from build123d import *

# Parameters (mm, degrees)
ESQUISSE1_R             = 8
BOSS_EXTRU_1_DEPTH      = 47.9
ESQUISSE2_R             = 4
BOSS_EXTRU_2_DEPTH      = 2.8
ESQUISSE3_R             = 2
BOSS_EXTRU_3_DEPTH      = 10
ESQUISSE5_W             = 4
ESQUISSE5_H             = 8
ENL_V_MAT_EXTRU_1_DEPTH = 10
BOSS_EXTRU_4_START      = 1.5
ESQUISSE6_R             = 4
BOSS_EXTRU_4_DEPTH      = 1.5
ESQUISSE7_R             = 1
ENL_V_MAT_EXTRU_2_DEPTH = 6


with BuildPart() as part:
    # Esquisse1 → Boss.-Extru.1 (new body)
    with BuildSketch(Plane.XY):
        Circle(ESQUISSE1_R)
    extrude(amount=BOSS_EXTRU_1_DEPTH)

    # Esquisse2 → Boss.-Extru.2 (add)
    with BuildSketch(Plane.XY.offset(47.9)):
        Circle(ESQUISSE2_R)
    extrude(amount=BOSS_EXTRU_2_DEPTH)

    # Esquisse3 → Boss.-Extru.3 (add)
    with BuildSketch(Plane.XY.offset(50.7)):
        Circle(ESQUISSE3_R)
    extrude(amount=BOSS_EXTRU_3_DEPTH)

    # Esquisse5 → Enlèv. mat.-Extru.1 (cut)
    with BuildSketch(Plane(origin=(0, 1, 0), x_dir=(1, 0, 0), z_dir=(0, 1, 0))):
        with Locations((0, -56.7)):
            Rectangle(ESQUISSE5_W, ESQUISSE5_H)
    extrude(amount=ENL_V_MAT_EXTRU_1_DEPTH, mode=Mode.SUBTRACT)

    # Esquisse6 → Boss.-Extru.4 (add)
    with BuildSketch(Plane(origin=(0, 0, 0), x_dir=(-1, 0, 0), z_dir=(0, 0, -1)).offset(BOSS_EXTRU_4_START)):
        with Locations(Location((0, 0, 0), (0, 0, 180))):
            Circle(ESQUISSE6_R)
    extrude(amount=-BOSS_EXTRU_4_DEPTH)

    # Esquisse7 → Enlèv. mat.-Extru.2 (cut)
    with BuildSketch(Plane.XY.offset(47.9)):
        with Locations((6, 0)):
            Circle(ESQUISSE7_R)
        with Locations((-6, 0)):
            Circle(ESQUISSE7_R)
    extrude(amount=-ENL_V_MAT_EXTRU_2_DEPTH, mode=Mode.SUBTRACT)


solid = part.part
Geometry check sheet. Reference: the model listing, model coordinates, mm. A direction names the side the tool comes from. Coordinates: 2 decimals unless noted, no trailing zeros. Order: outer loops, then holes, each group sorted by start corner. A loop starts at its lowest first (then second) coordinate and runs counter-clockwise, first axis right, second up. Notation, with made-up numbers: (15.25, 16.5) -> (21.25, 16.5) arc R18 cw to (21.25, 32.5) -> close; hole circle Ø11 at (39, -28.75). An arc over 180 degrees is marked (long way). Use a Markdown table: item, result. Add a question column.
1. Cross-section at A-A (x = 0). Enter the section's corners in (y, z), and give its area (3 significant figures).
2. Go/stop test with flat-tipped pins: pin 1 Ø2.5 at (x, y) = (-6, 0) entering from -Z; pin 2 Ø1.6 at (x, y) = (6, -0.5) entering from +Z; pin 3 Ø4 at (y, z) = (-2.5, 45) entering from -X. Record where each tip stops, or that it passes through.
3. Set-up check for faces 1 (the face through (-4, -2, 0)), 2 (the face through (-0.867, -3.905, 49.28)), 3 (the face through (0, 1, 57)): record each of +Z, -Z, +X, -X, +Y, -Y from which the full face is reachable in a straight line by a thin tool's end or side.
4. Material ranges on L1, parallel to X at y = -0.25, z = 8; L2, parallel to Y at x = -6, z = 46.3; L3, parallel to Z at x = -2, y = -3, recorded low to high.
5. Cross-section at B-B (y = 0). Enter the section's corners in (x, z), and give its area (3 significant figures).
6. Cross-section at D-D (z = 30.5). Enter the section's corners in (x, y), and give its area (3 significant figures).
7. Cross-section at C-C (z = 44.5). Enter the section's corners in (x, y), and give its area (3 significant figures).
8. Mould release check, pull along Y, two halves, no side actions. Record for faces 4 (the face through (-1.73, -7.81, 23.61)), 5 (the face through (-6.8, -0.6, 44.9)), 6 (the face through (0, 0, 60.7)): pulls with the +Y half, pulls with the -Y half, needs draft (parallel to the pull), parting line crosses it, or undercut.
Filled sheet:
| question | item | result |
|---|---|---|
| 1 | outline | (-8, 0) -> (-4, 0) -> (-4, -1.5) -> (4, -1.5) -> (4, 0) -> (8, 0) -> (8, 47.9) -> (4, 47.9) -> (4, 50.7) -> (2, 50.7) -> (2, 52.7) -> (1, 52.7) -> (1, 60.7) -> (-2, 60.7) -> (-2, 50.7) -> (-4, 50.7) -> (-4, 47.9) -> (-8, 47.9) -> close |
| 1 | area | 833 mm2 |
| 2 | pin 1 | z = 0 |
| 2 | pin 2 | z = 47.9 |
| 2 | pin 3 | x = -7.98 |
| 3 | face 1 | -Z |
| 3 | face 2 | +Z |
| 3 | face 3 | +Z, +X, -X, +Y |
| 4 | L1 | -8 to 8 |
| 4 | L2 | -5.29 to -1, 1 to 5.29 |
| 4 | L3 | -1.5 to 50.7 |
| 5 | outline | (-8, 0) -> (-4, 0) -> (-4, -1.5) -> (4, -1.5) -> (4, 0) -> (8, 0) -> (8, 47.9) -> (7, 47.9) -> (7, 41.9) -> (5, 41.9) -> (5, 47.9) -> (4, 47.9) -> (4, 50.7) -> (2, 50.7) -> (2, 60.7) -> (-2, 60.7) -> (-2, 50.7) -> (-4, 50.7) -> (-4, 47.9) -> (-5, 47.9) -> (-5, 41.9) -> (-7, 41.9) -> (-7, 47.9) -> (-8, 47.9) -> close |
| 5 | area | 817 mm2 |
| 6 | outline | circle Ø16 at (0, 0) |
| 6 | area | 201 mm2 |
| 7 | outline | circle Ø16 at (0, 0); hole circle Ø2 at (-6, 0); hole circle Ø2 at (6, 0) |
| 7 | area | 195 mm2 |
| 8 | face 4 | parting line crosses it |
| 8 | face 5 | undercut |
| 8 | face 6 | needs draft |
